For this review, use the dimensioned drawing (mm, ordinates from the lowest corner) and the shaded views. A direction names the side the tool comes from. Coordinates: 2 decimals unless noted, no trailing zeros. Loops run counter-clockwise (first coordinate to the right, second up) from the corner with the lowest first, then second, coordinate; pieces in that order, holes last. Notation, with made-up numbers: M 68.5,16 L 119.5,16 A22 ccw 119.5,28 Z; hole C 32,22.25 d9. An arc over 180 degrees is marked long. Write item = value, one per line.
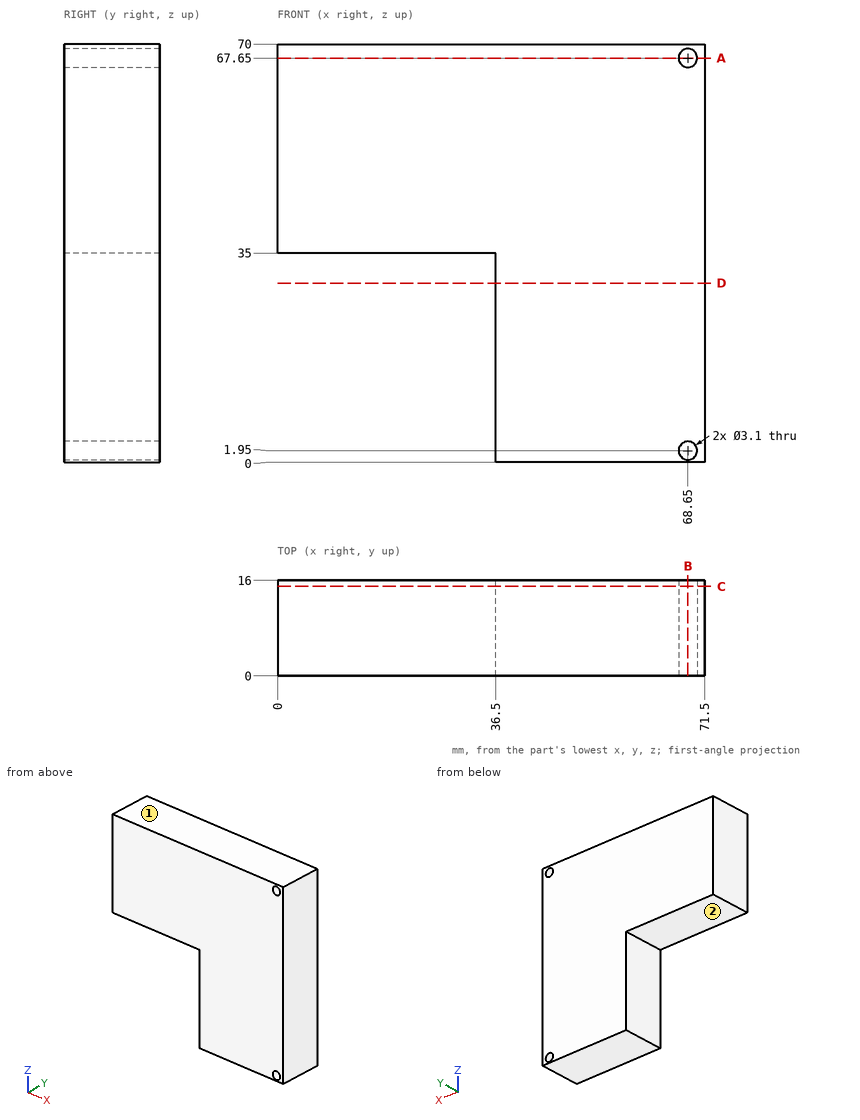
Q1. Add section A-A (z = 67.65). Write out the cut boundary in (x, y), and give its area (3 significant figures).
Solved:
outline = M 0,0 L 67.1,0 L 67.1,16 L 0,16 Z; M 70.2,0 L 71.5,0 L 71.5,16 L 70.2,16 Z
area = 1,090 mm²
Q2. Add section D-D (z = 30). Write out the cut boundary in (x, y), and give its area (3 significant figures).
Solved:
outline = M 36.5,0 L 71.5,0 L 71.5,16 L 36.5,16 Z
area = 560 mm²
Q3. For line 1 along Z through (x, y) = (68.65, 3.75); line 2 along X through (y, z) = (7.75, 67.65); line 3 along X through (y, z) = (9, 1.95), list the stretches that pass through material, from the lowest coordinate up.
Solved:
line_1 = 0 to 0.4, 3.5 to 66.1, 69.2 to 70
line_2 = 0 to 67.1, 70.2 to 71.5
line_3 = 36.5 to 67.1, 70.2 to 71.5
Q4. Add section B-B (x = 68.65). Write out the cut boundary in (y, z), and give its area (3 significant figures).
Solved:
outline = M 0,0 L 16,0 L 16,0.4 L 0,0.4 Z; M 0,3.5 L 16,3.5 L 16,66.1 L 0,66.1 Z; M 0,69.2 L 16,69.2 L 16,70 L 0,70 Z
area = 1,020 mm²
Q5. Machinability: for the marked faces 1 and 2, which of the approach directions +Z, -Z, +X, -X, +Y, -Y give a long, thin tool a straight path to every point of the face, cutting with its end or side? Answer none if there is none.
Solved:
face_1 = +Z, +X, -X, +Y, -Y
face_2 = -Z, -X, +Y, -Y
Q6. Add section C-C (y = 15). Write out the cut boundary in (x, z), and give its area (3 significant figures).
Solved:
outline = M 0,35 L 36.5,35 L 36.5,0 L 71.5,0 L 71.5,70 L 0,70 Z; hole C 68.65,1.95 d3.1; hole C 68.65,67.65 d3.1
area = 3,710 mm²
